Geometry: final body of the model. Coordinates: model frame, mm. Give positions to 0.01 mm unless a question says otherwise; leave off trailing zeros. Order: outer loops, then holes, each group sorted by start corner. A loop starts at its lowest first (then second) coordinate and runs counter-clockwise, first axis right, second up. Notation, with made-up numbers: (85.25, 81) -> (134.25, 81) arc R18 ccw to (134.25, 103) -> close; hole circle Ø7 at (85.5, 28). An arc over 180 degrees is marked (long way). One line per question, with ' | ' between items.
Autodesk Inventor part; units mm, degrees
ref_plane "YZ Plane" through (0, 0, 0) normal (1, 0, 0) x (0, 1, 0)
ref_plane "XZ Plane" through (0, 0, 0) normal (0, 1, 0) x (-1, 0, 0)
ref_plane "XY Plane" through (0, 0, 0) normal (0, 0, 1) x (1, 0, 0)
sketch "Sketch1" plane through (0, 0, 0) normal (0, 0, 1) x (1, 0, 0)
  line L0 (-65, -65) -> (65, -65)
  line L1 (65, -65) -> (65, 65)
  line L2 (65, 65) -> (-65, 65)
  line L3 (-65, 65) -> (-65, -65)
  line L4 (-65, -65) -> (65, 65) construction
  line L5 (65, -65) -> (-65, 65) construction
  point P0 (0, 0)
  dimension "d0" = 130
  dimension "d1" = 130
extrude "Extrusion1" add sketch "Sketch1" along normal blind 20
fillet "Fillet1" radius 8 4 edges at (65, -65, 10) (65, 65, 10) (-65, -65, 10) (-65, 65, 10)
sketch "Sketch2" plane through (0, 0, 20) normal (0, 0, 1) x (1, 0, 0)
  circle A0 centre (0, 0) radius 31.325
  dimension "d7" = 62.65
extrude "Extrusion2" cut sketch "Sketch2" against normal blind 10
1) Contact query for a flat-ended pin moving along its axis: pin 1 Ø1 at (x, y) = (1, -24) entering from +Z. Output: stop coordinate, or through.
Check result:
pin 1: stops at z = 10
2) Pull-direction query (Y, two-part tool) for faces 1 (the cylindrical face through (-62.594, 62.719, 10.14)), 2 (the cylindrical face through (-24.86, -19.06, 15.07)), 3 (the flat face through (0, 0, 10)), 4 (the flat face through (-30, 15, 20)); classes: +Y half, -Y half, draft (parallel to the pull), parting line (faces both ways), or undercut.
Check result:
face 1: +Y half | face 2: undercut | face 3: undercut | face 4: draft
3) Material intervals for probe 1 along Y at (x, z) = (0, 15.25) (3 decimals); probe 2 along Y at (x, z) = (-22, 19); probe 3 along Z at (x, y) = (-30, -3), sorted ascending. Write a range as from..to.
Check result:
probe 1: y = -65..-31.325, 31.325..65 | probe 2: y = -65..-22.3, 22.3..65 | probe 3: z = 0..10
4) Section A-A on z = 17. Return loops of the section in (x, y) (3 decimals).
Check result:
outline: (-65, -57) arc R8 ccw to (-57, -65) -> (57, -65) arc R8 ccw to (65, -57) -> (65, 57) arc R8 ccw to (57, 65) -> (-57, 65) arc R8 ccw to (-65, 57) -> close; hole circle Ø62.65 at (0, 0)
5) Section B-B on y = 0. Return loops of the section in (x, z) (3 decimals).
Check result:
outline: (-65, 0) -> (65, 0) -> (65, 20) -> (31.325, 20) -> (31.325, 10) -> (-31.325, 10) -> (-31.325, 20) -> (-65, 20) -> close
